```python
from build123d import *

# Parameters (mm, degrees)
SKETCH1_W          = 223
SKETCH1_H          = 175
SKETCH1_R          = 3.25
BASE_FLANGE1_DEPTH = 8
SKETCH2_R          = 5.5
CUT_EXTRUDE1_DEPTH = 142.959501267


# Sheet-metal steps are written as plain solids
with BuildPart() as part:
    # Sketch1 → Base-Flange1 (new body)
    with BuildSketch(Plane.XY):
        Rectangle(SKETCH1_W, SKETCH1_H)
        with Locations((15, 9.9)):
            Circle(SKETCH1_R, mode=Mode.SUBTRACT)
        with Locations((-15, 9.9)):
            Circle(SKETCH1_R, mode=Mode.SUBTRACT)
        with Locations((-15, -50.1)):
            Circle(SKETCH1_R, mode=Mode.SUBTRACT)
        with Locations((15, -50.1)):
            Circle(SKETCH1_R, mode=Mode.SUBTRACT)
    extrude(amount=-BASE_FLANGE1_DEPTH)

    # Sketch2 → Cut-Extrude1 (cut, through all)
    with BuildSketch(Plane.XY):
        with Locations((-96.5, 72.5)):
            Circle(SKETCH2_R)
        with Locations((-96.5, 37.5)):
            Circle(SKETCH2_R)
        with Locations(Location((96.5, 37.5, 0), (0, 0, 180))):
            Circle(SKETCH2_R)
        with Locations(Location((96.5, 72.5, 0), (0, 0, 180))):
            Circle(SKETCH2_R)
    extrude(amount=-CUT_EXTRUDE1_DEPTH, mode=Mode.SUBTRACT)


solid = part.part
```
For this review, take the finished solid that the model builds, in its own axes (mm). Round coordinates to 2 decimals unless told otherwise and drop trailing zeros. Loops run counter-clockwise (first coordinate to the right, second up) from the corner with the lowest first, then second, coordinate; pieces in that order, holes last.
Q1. Insertion check: pin 1 Ø3 at (x, y) = (85.5, -55.5) entering from +Z; pin 2 Ø4 at (x, y) = (15, -50.1) entering from +Z. Each pin has a flat end and moves straight along its axis. Give the tip position at first contact, or say it passes through.
Result sheet:
pin 1: stops at z = 0
pin 2: passes through
Q2. Add section B-B on x = -96.5. Write out the cut boundary in (y, z), plus the area to 3 significant figures.
Result sheet:
outline: (-87.5, -8) - (32, -8) - (32, 0) - (-87.5, 0) - close; (43, -8) - (67, -8) - (67, 0) - (43, 0) - close; (78, -8) - (87.5, -8) - (87.5, 0) - (78, 0) - close
area: 1,220 mm2
Q3. Add section A-A on y = 9.9. Write out the cut boundary in (x, z), plus the area to 3 significant figures.
Result sheet:
outline: (-111.5, -8) - (-18.25, -8) - (-18.25, 0) - (-111.5, 0) - close; (-11.75, -8) - (11.75, -8) - (11.75, 0) - (-11.75, 0) - close; (18.25, -8) - (111.5, -8) - (111.5, 0) - (18.25, 0) - close
area: 1,680 mm2
Q4. To check wall thickness, follow line 1 along Y through (x, z) = (-96.5, -5.5); line 2 along Y through (x, z) = (-16.5, -2.25). State the ranges of each line that lie inside material, in increasing order.
Result sheet:
line 1: y = -87.5 to 32, 43 to 67, 78 to 87.5
line 2: y = -87.5 to -52.98, -47.22 to 7.02, 12.78 to 87.5
Q5. Mouldability with a two-part tool opening along X and no side actions: class faces 1 (the face through (12.605, 12.097, -3.944)), 2 (the face through (111.5, -1, -4)), 3 (the face through (-17.395, 12.097, -3.944)), 4 (the face through (-2, 1, 0)) as +X half, -X half, draft (parallel to the pull), parting line (faces both ways), or undercut.
Result sheet:
face 1: undercut
face 2: +X half
face 3: undercut
face 4: draft
